Print and shaded views of the part. All mm, measured from the part's lowest x, y and z. A direction names the side the tool comes from. Coordinates: 2 decimals unless noted, no trailing zeros. Order: outer loops, then holes, each group sorted by start corner. A loop starts at its lowest first (then second) coordinate and runs counter-clockwise, first axis right, second up. Notation, with made-up numbers: (-33.5, -2) - (-15.5, -2) arc R31 ccw to (-15.5, 37) - close; hole circle Ø7 at (5.25, -34). An arc over 180 degrees is marked (long way). Write each question's results on one line, items separated by ' | '.
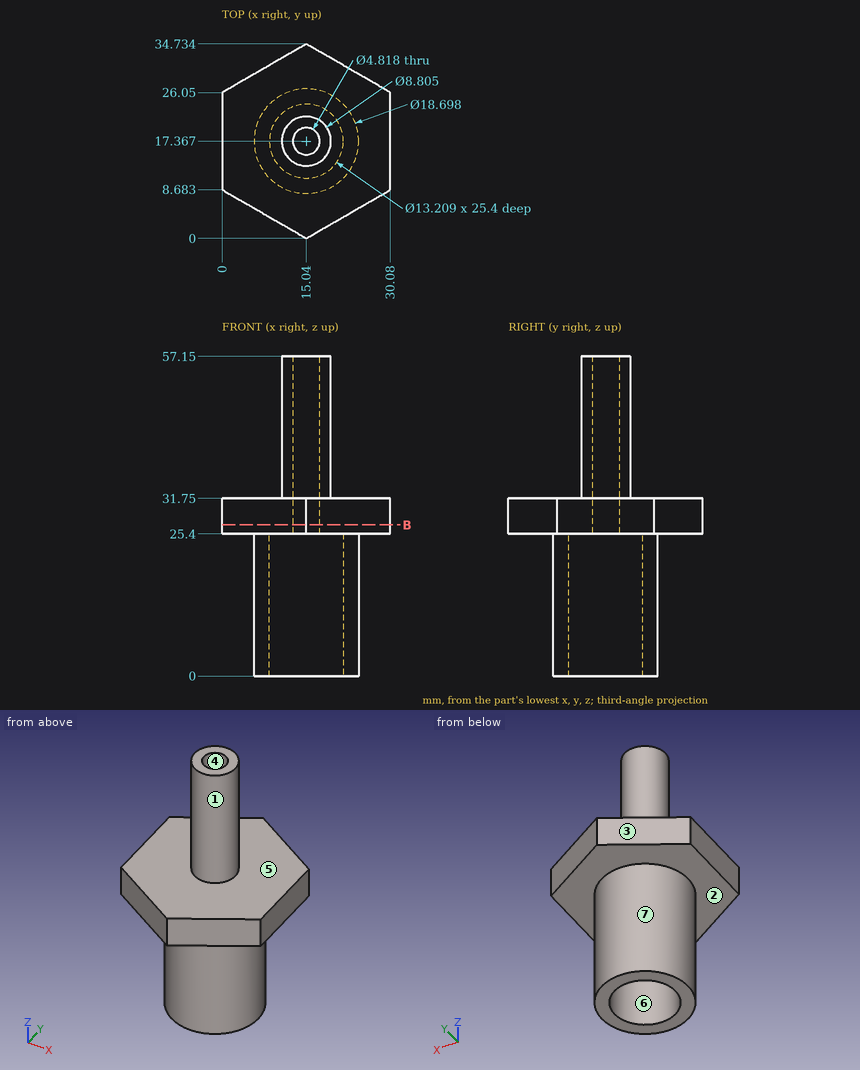
1. Two-plate mould, pull along Y, no slides. Class the marked faces 4, 5, 6 and 7: +Y half, -Y half, draft (parallel to the pull), parting line (faces both ways), or undercut.
Solved:
face 4: undercut | face 5: draft | face 6: undercut | face 7: parting line
2. Probe line 1 (Z direction, x = 5, y = 20); line 2 (Y direction, x = 17, z = 32) (1 decimal); line 3 (X direction, y = 16, z = 39.5) (1 decimal). List the from-to ranges inside material, lowest first.
Solved:
line 1: z = 25.4 to 31.75 | line 2: y = 13.4 to 16, 18.8 to 21.3 | line 3: x = 10.9 to 13.1, 17 to 19.2
3. Band-saw the part on B-B on z = 27. Give the cut face in (x, y), then the cut area to 3 significant figures.
Solved:
outline: (0, 8.68) - (15.04, 0) - (30.08, 8.68) - (30.08, 26.05) - (15.04, 34.73) - (0, 26.05) - close; hole circle Ø4.82 at (15.04, 17.37) | area: 765 mm2
4. Drop flat-ended pins along their axis: pin 1 Ø8 at (x, z) = (21, 7) entering from +Y; pin 2 Ø8 at (x, y) = (6, 6) entering from -Z; pin 3 Ø5 at (x, y) = (8.5, 21) entering from +Z. Give the stop position or say it passes through.
Solved:
pin 1: stops at y = 26.51 | pin 2: stops at z = 25.4 | pin 3: stops at z = 31.75
5. Tool access for the marked faces 1, 2 and 3: list every direction of +Z, -Z, +X, -X, +Y, -Y with a clear straight run to the whole face (end or side of a thin tool).
Solved:
face 1: +Z | face 2: -Z | face 3: +Z, -Z, -X, +Y
